Part model, mm, in its own coordinate system. A direction names the side the tool comes from. Give positions to 0.01 mm unless a question says otherwise; leave off trailing zeros. Write each loop counter-clockwise with the first axis right and the second up, starting at its lowest first coordinate (ties: lowest second). Pieces come first, ordered by that corner, then holes. Notation, with made-up numbers: M 12,-15 L 18,-15 A29 ccw 18,13 Z; hole C -8.5,55.25 d6. An arc over 180 degrees is marked long. Use a Markdown table: item, result.
Solid Edge part; units mm, degrees
sketch "Sketch1" plane through (0, 0, 0) normal (0, -1, 0) x (1, 0, 0)
  line L0 (-14, -12) -> (14, -12)
  line L1 (14, -12) -> (14, 12)
  line L2 (14, 12) -> (-14, 12)
  line L3 (-14, 12) -> (-14, -12)
  dimension "D1" = 14
  dimension "D2" = 14
extrude "Protrusion1" add sketch "Sketch1" along normal mid plane 5
sketch "Sketch2" plane through (0, -2.5, 0) normal (0, -1, 0) x (1, 0, 0)
  circle A0 centre (0, 12) radius 12
extrude "Extrusionsausschnitt_1" cut sketch "Sketch2" against normal blind 221
hole "Bohrung_1" at (-10, 0, -12) direction (0, 0, 1) diameter 3.5 depth 8
hole "Hole1" at (10, 0, -12) direction (0, 0, 1) diameter 3.5 depth 8
mirror "Mirror1" about plane through (-13.5, 0, 12) normal (0, 0, 1) of "Protrusion1", "Extrusionsausschnitt_1"
sketch "Sketch3" plane through (0, 0, 36) normal (0, 0, 1) x (1, 0, 0)
  line L0 (-14, 2.5) -> (14, 2.5)
  line L1 (14, 2.5) -> (14, -2.5)
  line L2 (14, -2.5) -> (-14, -2.5)
  line L3 (-14, -2.5) -> (-14, 2.5)
extrude "Extrusionsausprägung_3" add sketch "Sketch3" along normal blind 6
hole "Bohrung_5" at (-10, 0, 42) direction (0, 0, -1) diameter 3.5 depth 8
hole "Hole2" at (10, 0, 42) direction (0, 0, -1) diameter 3.5 depth 8
properties material "Aluminiumlegierung:3.0205, Al 99.0, EN-AW 1200"
1. Drop flat-ended pins along their axis: P1, Ø3, axis at x = -10, y = 0, coming from the -Z side; P2, Ø6, axis at x = 7, z = 15, coming from the +Y side; P3, Ø1, axis at x = 10, y = 0.5, coming from the +Z side. Give the stop position or say it passes through.
Findings below:
| item | result |
|---|---|
| P1 | z = -4 |
| P2 | through |
| P3 | z = 34 |
2. Cut at A-A, the plane y = 0. Give the cut face in (x, z).
Findings below:
| item | result |
|---|---|
| outline | M -14,-12 L -11.75,-12 L -11.75,-4 L -8.25,-4 L -8.25,-12 L 8.25,-12 L 8.25,-4 L 11.75,-4 L 11.75,-12 L 14,-12 L 14,42 L 11.75,42 L 11.75,34 L 8.25,34 L 8.25,42 L -8.25,42 L -8.25,34 L -11.75,34 L -11.75,42 L -14,42 Z; hole C 0,12 d24 |
3. Cut at C-C, the plane z = 12. Give the cut face in (x, y).
Findings below:
| item | result |
|---|---|
| outline | M -14,-2.5 L -12,-2.5 L -12,2.5 L -14,2.5 Z; M 12,-2.5 L 14,-2.5 L 14,2.5 L 12,2.5 Z |
4. Tool access for faces 5 (the flat face through (-10, 0, 34)), 6 (the flat face through (10, -2.5, 21)), 7 (the flat face through (-10, 0, -4)): list every direction of +Z, -Z, +X, -X, +Y, -Y with a clear straight run to the whole face (end or side of a thin tool).
Findings below:
| item | result |
|---|---|
| face 5 | +Z |
| face 6 | +Z, -Z, +X, -X, -Y |
| face 7 | -Z |
5. Cut at D-D, the plane z = -8. Give the cut face in (x, y), then the cut area to 3 significant figures.
Findings below:
| item | result |
|---|---|
| outline | M -14,-2.5 L 14,-2.5 L 14,2.5 L -14,2.5 Z; hole C -10,0 d3.5; hole C 10,0 d3.5 |
| area | 121 mm2 |
6. Two-plate mould, pull along Z, no slides. Class faces 1 (the flat face through (-14, 0, 15)), 2 (the flat face through (0, 0, 42)), 3 (the cylindrical face through (-8.844, -0.035, 20.11)), 4 (the flat face through (0, 0, -12)): released by +Z, released by -Z, zero draft, split by the parting line, or undercut.
Findings below:
| item | result |
|---|---|
| face 1 | zero draft |
| face 2 | released by +Z |
| face 3 | undercut |
| face 4 | released by -Z |
7. Cut at B-B, the plane x = 0. Give the cut face in (y, z), then the cut area to 3 significant figures.
Findings below:
| item | result |
|---|---|
| outline | M -2.5,-12 L 2.5,-12 L 2.5,0 L -2.5,0 Z; M -2.5,24 L 2.5,24 L 2.5,42 L -2.5,42 Z |
| area | 150 mm2 |
8. Drill centre lines: L1, parallel to X at y = 0, z = -6.5; L2, parallel to X at y = 0.5, z = 12; L3, parallel to X at y = 1.6, z = 37.5. Where is each one in solid material? Low to high.
Findings below:
| item | result |
|---|---|
| L1 | -14 to -11.75, -8.25 to 8.25, 11.75 to 14 |
| L2 | -14 to -12, 12 to 14 |
| L3 | -14 to -10.71, -9.29 to 9.29, 10.71 to 14 |
